Input: part model. Units: mm. Frame: model coordinates. Face numbers are marked on the shaded views. A direction names the side the tool comes from. Coordinates: 2 decimals unless noted, no trailing zeros. Loops run counter-clockwise (first coordinate to the right, second up) from the corner with the lowest first, then second, coordinate; pieces in that order, holes last. Notation, with made-up numbers: (-24, 26.25) -> (-14, 26.25) arc R26 ccw to (-14, 45.25) -> close; hole circle Ø10 at (-10.5, 27.25). An arc over 180 degrees is marked (long way). Answer as a JSON object with one key per item and string values.
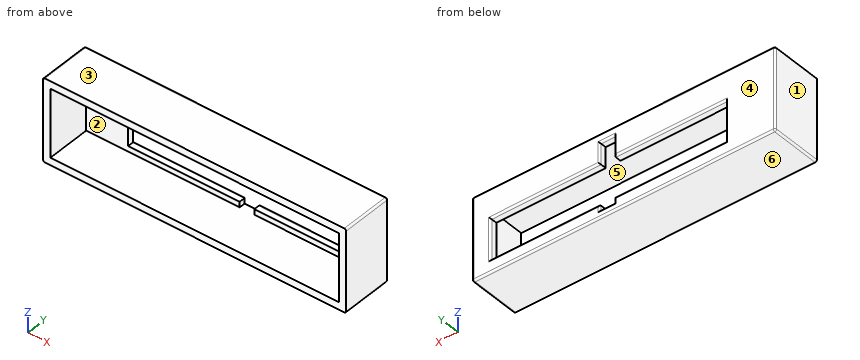
from build123d import *

# Parameters (mm, degrees)
SKETCH1_W           = 209.55
SKETCH1_H           = 57.15
BOSS_EXTRUDE1_DEPTH = 5.08
SKETCH2_W           = 209.55
SKETCH2_H           = 57.15
SKETCH2_W_2         = 199.39
SKETCH2_H_2         = 46.99
BOSS_EXTRUDE2_DEPTH = 30.48
CUT_EXTRUDE2_REACH  = 117.837
FILLET1_R           = 1.27


with BuildPart() as part:
    # Sketch1 → Boss-Extrude1 (new body)
    with BuildSketch(Plane(origin=(0, 0, 0), x_dir=(1, 0, 0), z_dir=(0, 1, 0))):
        with Locations((0, -5.715)):
            Rectangle(SKETCH1_W, SKETCH1_H)
    extrude(amount=BOSS_EXTRUDE1_DEPTH)

    # Sketch2 → Boss-Extrude2 (add)
    with BuildSketch(Plane.XZ):
        with Locations((0, 5.715)):
            Rectangle(SKETCH2_W, SKETCH2_H)
        with Locations((0, 5.715)):
            Rectangle(SKETCH2_W_2, SKETCH2_H_2, mode=Mode.SUBTRACT)
    extrude(amount=BOSS_EXTRUDE2_DEPTH)

    # Sketch3 → Cut-Extrude2 (cut, up to next)
    with BuildSketch(Plane(origin=(0, 5.08, 0), x_dir=(1, 0, 0), z_dir=(0, 1, 0)), mode=Mode.PRIVATE) as cut_extrude2_sk1:
        Polygon((6.35, 13.97), (-70.668502474, 13.97), (-70.668502474, -13.97), (6.35, -13.97), (6.35, -28.17903858), (16.51, -28.17903858), (16.51, -13.97), (92.086948761, -13.97), (92.086948761, 13.97), (16.51, 13.97), (16.51, 17.78), (6.35, 17.78), align=None)
    cut_extrude2_tool1 = extrude(cut_extrude2_sk1.sketch, amount=-CUT_EXTRUDE2_REACH, mode=Mode.PRIVATE) & part.part
    add(cut_extrude2_tool1.solids().sort_by_distance((10.737118, 5.08, 0.513245))[0], mode=Mode.SUBTRACT)

    # Fillet1
    fillet1_edges = [part.edges().sort_by_distance(p)[0] for p in [
        (-104.775, 5.08, 5.715),
        (0, 5.08, 34.29),
        (92.086948761, 5.08, 0),
        (-70.668502474, 5.08, 0),
        (-32.159251237, 5.08, 13.97),
        (6.35, 5.08, 21.07451929),
        (11.43, 5.08, 28.17903858),
        (54.29847438, 5.08, 13.97),
        (104.775, 5.08, 5.715),
        (16.51, 5.08, -15.875),
        (-32.159251237, 5.08, -13.97),
        (54.29847438, 5.08, -13.97),
        (16.51, 5.08, 21.07451929),
        (11.43, 5.08, -17.78),
        (6.35, 5.08, -15.875),
        (104.775, -12.7, 34.29),
        (-104.775, -12.7, 34.29),
        (-104.775, -12.7, -22.86),
        (104.775, -12.7, -22.86),
        (0, 5.08, -22.86),
    ]]
    fillet(fillet1_edges, radius=FILLET1_R)


solid = part.part
1. Mould query, pull axis Z, two halves, no side actions, for the marked faces 3, 4, 5 and 6. Classes: pulls with the +Z half, pulls with the -Z half, needs draft (parallel to the pull), parting line crosses it, or undercut.
Reply:
{"face 3": "pulls with the +Z half", "face 4": "needs draft", "face 5": "undercut", "face 6": "pulls with the -Z half"}
2. Access query for the marked faces 1 and 2. Directions: +Z, -Z, +X, -X, +Y, -Y. A direction counts if a zero-diameter tool reaches every point of the face in a straight line with its end or side. Return the directions, or none.
Reply:
{"face 1": "+Z, -Z, -X, +Y, -Y", "face 2": "-Y"}
3. Section query A-A (x = -20.5). Return loops of the section in (y, z).
Reply:
{"outline": "(-30.48, -22.86) -> (3.81, -22.86) arc R1.27 ccw to (5.08, -21.59) -> (5.08, -15.24) arc R1.27 ccw to (3.81, -13.97) -> (0, -13.97) -> (0, -17.78) -> (-30.48, -17.78) -> close; (-30.48, 29.21) -> (0, 29.21) -> (0, 13.97) -> (3.81, 13.97) arc R1.27 ccw to (5.08, 15.24) -> (5.08, 33.02) arc R1.27 ccw to (3.81, 34.29) -> (-30.48, 34.29) -> close"}
4. Section query D-D (x = -91.5). Return loops of the section in (y, z), plus the area to 3 significant figures.
Reply:
{"outline": "(-30.48, -22.86) -> (3.81, -22.86) arc R1.27 ccw to (5.08, -21.59) -> (5.08, 33.02) arc R1.27 ccw to (3.81, 34.29) -> (-30.48, 34.29) -> (-30.48, 29.21) -> (0, 29.21) -> (0, -17.78) -> (-30.48, -17.78) -> close", "area": "599 mm2"}
5. Pin query (flat end, axial travel): P1, Ø1.5, axis at x = 49.5, z = 18, coming from the -Y side; P2, Ø3, axis at x = -4, z = 11.5, coming from the -Y side. Return the tip coordinate at first contact, or that it passes through.
Reply:
{"P1": "stops at y = 0", "P2": "passes through"}
6. Line query: line 1 along Z through (x, y) = (49.5, -26.5); line 2 along X through (y, z) = (-27.5, -2) (3 decimals); line 3 along Z through (x, y) = (-55, 1.5). Output: solid intervals per line, ascending.
Reply:
{"line 1": "z = -22.86 to -17.78, 29.21 to 34.29", "line 2": "x = -104.775 to -99.695, 99.695 to 104.775", "line 3": "z = -22.86 to -13.97, 13.97 to 34.29"}
7. Section query C-C (y = -16). Return loops of the section in (x, z) (3 decimals), plus the area to 3 significant figures.
Reply:
{"outline": "(-104.775, -21.59) arc R1.27 ccw to (-103.505, -22.86) -> (103.505, -22.86) arc R1.27 ccw to (104.775, -21.59) -> (104.775, 33.02) arc R1.27 ccw to (103.505, 34.29) -> (-103.505, 34.29) arc R1.27 ccw to (-104.775, 33.02) -> close; hole (-99.695, -17.78) -> (99.695, -17.78) -> (99.695, 29.21) -> (-99.695, 29.21) -> close", "area": "2,610 mm2"}
8. Section query B-B (z = 8). Return loops of the section in (x, y) (1 decimal), plus the area to 3 significant figures.
Reply:
{"outline": "(-104.8, -30.5) -> (-99.7, -30.5) -> (-99.7, 0) -> (-70.7, 0) -> (-70.7, 3.8) arc R1.3 ccw to (-71.9, 5.1) -> (-103.5, 5.1) arc R1.3 ccw to (-104.8, 3.8) -> close; (92.1, 0) -> (99.7, 0) -> (99.7, -30.5) -> (104.8, -30.5) -> (104.8, 3.8) arc R1.3 ccw to (103.5, 5.1) -> (93.4, 5.1) arc R1.3 ccw to (92.1, 3.8) -> close", "area": "546 mm2"}
